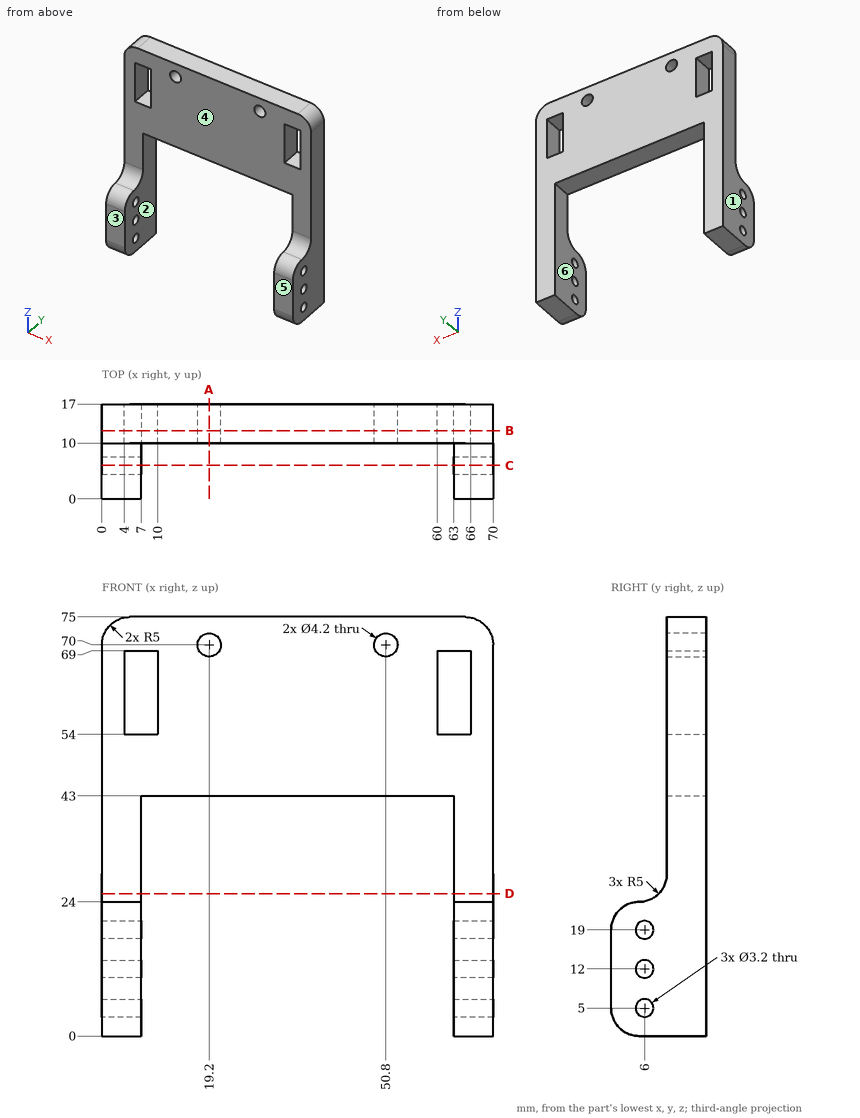
Geometry: see drawing. Coordinates: mm, zero at the bounding-box minimum. A direction names the side the tool comes from. Give positions to 0.01 mm unless a question says otherwise; leave off trailing zeros. Loops run counter-clockwise (first coordinate to the right, second up) from the corner with the lowest first, then second, coordinate; pieces in that order, holes last. Notation, with made-up numbers: (48.25, 24) - (105.25, 24) arc R25 ccw to (105.25, 48) - close; hole circle Ø3 at (21, -30.75). An arc over 180 degrees is marked (long way). One line per question, with ' | ' between items. Start each with the question number.
(1) Ray query, line 1 (X direction, y = 15.5, z = 63); line 2 (Y direction, x = 67, z = 5); line 3 (X direction, y = 11.5, z = 33). Return the intervals inside material, ascending. Write a range as from..to.
(2) Reachability of the marked faces 4, 5 and 6 from +Z, -Z, +X, -X, +Y, -Y: full face, straight path, thin tool, end or side. Return the list, or none.
(3) Section query B-B on y = 12.25. Return loops of the section in (x, z), then the cut area to 3 significant figures.
(4) Pull-direction query (X, two-part tool) for the marked faces 1, 2 and 3; classes: released by +X, released by -X, zero draft, split by the parting line, or undercut.
(5) Section query D-D on z = 25.5. Return loops of the section in (x, y).
(6) Section query A-A on x = 19.2. Return loops of the section in (y, z), then the cut area to 3 significant figures.
(7) Contact query for flat-ended pins moving along their axis: pin 1 (3 mm diameter, centred on y = 6, z = 12, fed in from +X); pin 2 (5 mm diameter, centred on x = 19.2, z = 70, fed in from -Y). Output: stop coordinate, or through.
(8) Section query C-C on y = 6. Count the separate pieces of the cut face and the enclosed holes in it, then the cut area to 3 significant figures.
The answers:
1) line 1: 0..4, 10..60, 66..70 | line 2: 0..4.4, 7.6..17 | line 3: 0..7, 63..70
2) face 4: +Z, +X, -X, -Y | face 5: +Z, -Z, +X, -X, -Y | face 6: -Z, +Y, -Y
3) outline: (0, 0) - (7, 0) - (7, 43) - (63, 43) - (63, 0) - (70, 0) - (70, 70) arc R5 ccw to (65, 75) - (5, 75) arc R5 ccw to (0, 70) - close; hole (4, 54) - (10, 54) - (10, 69) - (4, 69) - close; hole circle Ø4.2 at (19.2, 70); hole circle Ø4.2 at (50.8, 70); hole (60, 54) - (66, 54) - (66, 69) - (60, 69) - close | area: 2,620 mm2
4) face 1: released by -X | face 2: undercut | face 3: zero draft
5) outline: (0, 8.57) - (7, 8.57) - (7, 17) - (0, 17) - close; (63, 8.57) - (70, 8.57) - (70, 17) - (63, 17) - close
6) outline: (10, 43) - (17, 43) - (17, 67.9) - (10, 67.9) - close; (10, 72.1) - (17, 72.1) - (17, 75) - (10, 75) - close | area: 195 mm2
7) pin 1: through | pin 2: y = 10
8) separate pieces: 8 | enclosed holes: 0 | area: 203 mm2
